```python
from build123d import *

# Parameters (mm, degrees)
CUT_EXTRUDE1_REACH = 119.708
SKETCH2_R          = 11.58920475
FILLET1_R          = 2
CUT_EXTRUDE3_REACH = 123.601
CHAMFER1_SIZE      = 0.5


with BuildPart() as part:
    # Sketch1 → Revolve1 (revolve)
    with BuildSketch(Plane(origin=(0, 0, 0), x_dir=(0, 0, -1), z_dir=(1, 0, 0)), mode=Mode.PRIVATE) as revolve1_sk:
        Polygon((-17.414092448, 19), (20.585907552, 19), (20.585907552, 30.4), (5.221286802, 30.4), (5.221286802, 71.23775235), (18.385907552, 71.23775235), (18.385907552, 81.6785385), (-15.214092448, 81.6785385), (-15.214092448, 71.23775235), (-2.049471698, 71.23775235), (-2.049471698, 30.4), (-17.414092448, 30.4), align=None)
    revolve(revolve1_sk.sketch.rotate(Axis((0, 0, 17.414092448), (0, 0, -1)), 90), axis=Axis((0, 0, 17.414092448), (0, 0, -1)))

    # Sketch2 → Cut-Extrude1 (cut, up to next)
    with BuildSketch(Plane.XY.offset(2.049471698), mode=Mode.PRIVATE) as cut_extrude1_sk1:
        with Locations((0, 50.8188762)):
            Circle(SKETCH2_R)
    cut_extrude1_tool1 = extrude(cut_extrude1_sk1.sketch, amount=-CUT_EXTRUDE1_REACH, mode=Mode.PRIVATE) & part.part
    # Sketch2 → Cut-Extrude1 (cut, up to next)
    with BuildSketch(Plane.XY.offset(2.049471698), mode=Mode.PRIVATE) as cut_extrude1_sk2:
        with Locations((44.010437781, 25.4094381)):
            Circle(SKETCH2_R)
    cut_extrude1_tool2 = extrude(cut_extrude1_sk2.sketch, amount=-CUT_EXTRUDE1_REACH, mode=Mode.PRIVATE) & part.part
    # Sketch2 → Cut-Extrude1 (cut, up to next)
    with BuildSketch(Plane.XY.offset(2.049471698), mode=Mode.PRIVATE) as cut_extrude1_sk3:
        with Locations((44.010437781, -25.4094381)):
            Circle(SKETCH2_R)
    cut_extrude1_tool3 = extrude(cut_extrude1_sk3.sketch, amount=-CUT_EXTRUDE1_REACH, mode=Mode.PRIVATE) & part.part
    # Sketch2 → Cut-Extrude1 (cut, up to next)
    with BuildSketch(Plane.XY.offset(2.049471698), mode=Mode.PRIVATE) as cut_extrude1_sk4:
        with Locations((0, -50.8188762)):
            Circle(SKETCH2_R)
    cut_extrude1_tool4 = extrude(cut_extrude1_sk4.sketch, amount=-CUT_EXTRUDE1_REACH, mode=Mode.PRIVATE) & part.part
    # Sketch2 → Cut-Extrude1 (cut, up to next)
    with BuildSketch(Plane.XY.offset(2.049471698), mode=Mode.PRIVATE) as cut_extrude1_sk5:
        with Locations((-44.010437781, -25.4094381)):
            Circle(SKETCH2_R)
    cut_extrude1_tool5 = extrude(cut_extrude1_sk5.sketch, amount=-CUT_EXTRUDE1_REACH, mode=Mode.PRIVATE) & part.part
    # Sketch2 → Cut-Extrude1 (cut, up to next)
    with BuildSketch(Plane.XY.offset(2.049471698), mode=Mode.PRIVATE) as cut_extrude1_sk6:
        with Locations((-44.010437781, 25.4094381)):
            Circle(SKETCH2_R)
    cut_extrude1_tool6 = extrude(cut_extrude1_sk6.sketch, amount=-CUT_EXTRUDE1_REACH, mode=Mode.PRIVATE) & part.part
    add(cut_extrude1_tool1.solids().sort_by_distance((0, 50.818876, 2.049472))[0], mode=Mode.SUBTRACT)
    add(cut_extrude1_tool2.solids().sort_by_distance((44.010438, 25.409438, 2.049472))[0], mode=Mode.SUBTRACT)
    add(cut_extrude1_tool3.solids().sort_by_distance((44.010438, -25.409438, 2.049472))[0], mode=Mode.SUBTRACT)
    add(cut_extrude1_tool4.solids().sort_by_distance((0, -50.818876, 2.049472))[0], mode=Mode.SUBTRACT)
    add(cut_extrude1_tool5.solids().sort_by_distance((-44.010438, -25.409438, 2.049472))[0], mode=Mode.SUBTRACT)
    add(cut_extrude1_tool6.solids().sort_by_distance((-44.010438, 25.409438, 2.049472))[0], mode=Mode.SUBTRACT)

    # Fillet1
    fillet1_edges = [part.edges().sort_by_distance(p)[0] for p in [
        (-71.23775235, 0, 2.049471698),
        (-71.23775235, 0, -5.221286802),
        (-30.4, 0, -5.221286802),
        (-30.4, 0, 2.049471698),
    ]]
    fillet(fillet1_edges, radius=FILLET1_R)

    # Sketch4 → Cut-Extrude3 (cut, up to next)
    with BuildSketch(Plane.XY.offset(17.414092448), mode=Mode.PRIVATE) as cut_extrude3_sk1:
        with BuildLine():
            Line((-22.3, 5), (-22.3, -5))
            Line((-22.3, -5), (-18.33030278, -5))
            ThreePointArc((-18.33030278, -5), (-19, 0), (-18.33030278, 5))
            Line((-18.33030278, 5), (-22.3, 5))
        make_face()
    cut_extrude3_tool1 = extrude(cut_extrude3_sk1.sketch, amount=-CUT_EXTRUDE3_REACH, mode=Mode.PRIVATE) & part.part
    add(cut_extrude3_tool1.solids().sort_by_distance((-20.533552, 0, 17.414092))[0], mode=Mode.SUBTRACT)

    # Chamfer1
    chamfer1_edges = [part.edges().sort_by_distance(p)[0] for p in [
        (-81.6785385, 0, 15.214092448),
        (-81.6785385, 0, -18.385907552),
        (-30.4, 0, -20.585907552),
        (-30.4, 0, 17.414092448),
    ]]
    chamfer(chamfer1_edges, length=CHAMFER1_SIZE)


solid = part.part
```
Model file for the job. Use its own axes, mm. A direction names the side the tool comes from. Round coordinates to 2 decimals unless told otherwise and drop trailing zeros. Loops run counter-clockwise (first coordinate to the right, second up) from the corner with the lowest first, then second, coordinate; pieces in that order, holes last. Notation, with made-up numbers: M 41.5,10 L 92.5,10 A17 cw 92.5,38 Z; hole C 44.25,-9 d11. An arc over 180 degrees is marked long. Put each result on its own line as item: value. Start each with the question number.
Item 1: 3-axis set-ups, long thin cutter, end or side, ignore diameter. For faces 4 (the face through (-22.3, 0, -1)), 5 (the face through (-9.274, -70.632, 9.554)), 6 (the face through (-9.274, -70.632, -12.882)): which of +Z, -Z, +X, -X, +Y, -Y reach the whole face in a straight line?
Item 2: Drop flat-ended pins along their axis: P1, Ø2, axis at x = 16.5, z = -8.5, coming from the -Y side; P2, Ø18.5, axis at x = 0, y = 50.82, coming from the +Z side; P3, Ø1.2, axis at x = -19.5, z = 5.5, coming from the -Y side; P4, Ø12, axis at x = 10, z = -9.5, coming from the +Y side. Give the stop position or say it passes through.
Item 3: Cut at A-A (z = 11). List the corners of the cut face in (x, y), then the cut area to 3 significant figures.
Item 4: Drill centre lines: line 1 along Y through (x, z) = (0, 0); line 2 along Y through (x, z) = (0, 11); line 3 along Y through (x, z) = (45.5, 2). Where is each one in solid material? Low to high.
Item 5: Mould opens along X. For faces 1 (the face through (0, 72, -18.386)), 2 (the face through (28.996, -9.131, -13.564)), 3 (the face through (-64.817, 49.7, -1.358)) say: released by +X, released by -X, zero draft, split by the parting line, or undercut.
Item 6: Cut at B-B (x = 0). Give the number of separate pieces and of enclosed holes in the cut face, then the cut area to 3 significant figures.
Answer block:
1. face 4: +Z, -Z
1. face 5: +Z
1. face 6: -Z
2. P1: y = -80.19
2. P2: through
2. P3: y = -79.46
2. P4: y = 81.58
3. outline: C 0,0 d163.36; C 0,0 d60.8; hole C 0,0 d142.48; hole M -22.3,-5 L -18.33,-5 A19 ccw long -18.33,5 L -22.3,5 Z
3. area: 6,750 mm2
4. line 1: -81.68 to -62.41, -39.23 to -19, 19 to 39.23, 62.41 to 81.68
4. line 2: -81.68 to -71.24, -30.4 to -19, 19 to 30.4, 71.24 to 81.68
4. line 3: -67.83 to -36.9, -13.92 to 13.92, 36.9 to 67.83
5. face 1: zero draft
5. face 2: undercut
5. face 3: split by the parting line
6. separate pieces: 4
6. enclosed holes: 0
6. area: 1,830 mm2
